The listing builds one solid part. Answer for the finished solid, in the listing's coordinates (mm). A direction names the side the tool comes from. Give positions to 0.01 mm unless a question says otherwise; leave off trailing zeros. Order: outer loops, then holes, each group sorted by start corner. A loop starts at its lowest first (then second) coordinate and runs counter-clockwise, first axis right, second up. Notation, with made-up numbers: (7, 41.5) -> (53, 41.5) arc R29 cw to (53, 74.5) -> close; hole circle Ø7 at (11, -34). An arc over 180 degrees is marked (long way). Write item = value, one per line. Start each with the question number.
Autodesk Inventor part; units mm, degrees
ref_plane "YZ Plane" through (0, 0, 0) normal (1, 0, 0) x (0, 1, 0)
ref_plane "XZ Plane" through (0, 0, 0) normal (0, 1, 0) x (-1, 0, 0)
ref_plane "XY Plane" through (0, 0, 0) normal (0, 0, 1) x (1, 0, 0)
sketch "Sketch1" plane through (0, 0, 0) normal (0, 1, 0) x (-1, 0, 0)
  line L0 (0, 0) -> (11.43, 0)
  line L1 (11.43, 0) -> (11.43, -25.4)
  line L2 (11.43, -25.4) -> (0, -25.4)
  line L3 (0, -25.4) -> (0, 0)
  dimension "d0" = 11.43
  dimension "d1" = 25.4
extrude "Extrusion1" add sketch "Sketch1" along normal blind 10.16
sketch "Sketch2" plane through (0, 10.16, 0) normal (0, 1, 0) x (1, 0, 0)
  line L0 (0, 0) -> (0, 25.4)
  line L1 (0, 0) -> (-6.985, 0)
  line L2 (-6.985, 0) -> (-6.985, 4.6296)
  line L3 (-6.985, 4.6296) -> (0, 4.6296)
  line L4 (0, 4.6296) -> (0, 0)
  line L5 (-6.985, 0) -> (-8.8265, 0)
  line L6 (-8.8265, 0) -> (-8.8265, 15.875)
  line L7 (-8.8265, 15.875) -> (-6.985, 15.875)
  line L8 (-6.985, 15.875) -> (-6.985, 0)
  dimension "d4" = 6.985
  dimension "d5" = 1.8415
  dimension "d6" = 15.875
extrude "Extrusion2" cut sketch "Sketch2" against normal blind 12.7 contours L5 L6 L7 L8 L2
properties part number "PCB_Holder"
Item 1: A cutting plane is placed at B-B, the plane y = 4.25. Write down the section's boundary in (x, z) (1 decimal), plus the area to 3 significant figures.
Item 2: A cutting plane is placed at A-A, the plane z = -3.5. Write down the section's boundary in (x, y) (1 decimal), plus the area to 3 significant figures.
Item 3: Which of the six approach directions +Z, -Z, +X, -X, +Y, -Y give full straight-line access (tool end or side, diameter ignored) to faces 1 (the flat face through (-8, 5, -15.875)), 2 (the flat face through (-10, 5, 0))?
Item 4: The mould has two halves that part along X. Classify faces 3 (the flat face through (-8.826, 5, -8)), 4 (the flat face through (0, 5, -13)), 5 (the flat face through (-6, 10.16, -13)): +X half, -X half, draft (parallel to the pull), parting line (faces both ways), or undercut.
Item 5: Consider L1, parallel to X at y = 9.75, z = -2.5 (1 decimal); L2, parallel to Z at x = -7.5, y = 4.75 (3 decimals). Determine where each line is inside the solid, lowest interval first. Write a range as from..to.
Check values:
q1.outline = (-11.4, -25.4) -> (0, -25.4) -> (0, 0) -> (-7, 0) -> (-7, -15.9) -> (-8.8, -15.9) -> (-8.8, 0) -> (-11.4, 0) -> close
q1.area = 261 mm^2
q2.outline = (-11.4, 0) -> (-8.8, 0) -> (-8.8, 10.2) -> (-11.4, 10.2) -> close; (-7, 0) -> (0, 0) -> (0, 10.2) -> (-7, 10.2) -> close
q2.area = 97.4 mm^2
q3.face_1 = +Z, +Y, -Y
q3.face_2 = +Z, +X, -X, +Y, -Y
q4.face_3 = undercut
q4.face_4 = +X half
q4.face_5 = draft
q5.L1 = -11.4..-8.8, -7..0
q5.L2 = -25.4..-15.875
